The listing builds one solid part. Answer for the finished solid, in the listing's coordinates (mm). A direction names the side the tool comes from. Round coordinates to 2 decimals unless told otherwise and drop trailing zeros. Write each loop counter-clockwise with the first axis right and the second up, starting at its lowest first coordinate (ties: lowest second). Pieces come first, ordered by that corner, then holes.
Item 1: Each of these flat-tipped pins is pushed along its axis until it touches: pin 1 (8 mm diameter, centred on y = -8, z = 5, fed in from -X); pin 2 (1.5 mm diameter, centred on y = 12, z = 5, fed in from -X); pin 3 (6 mm diameter, centred on x = -1, z = 10, fed in from +Y) (3 decimals); pin 4 (4 mm diameter, centred on x = -11.5, z = 4, fed in from -Y). Where does it stop, or does it pass through?
Item 2: A tool of negligible diameter and unlimited length cuts with its end or side. For faces 5 (the face through (-5.474, 3.219, 12.522)), 6 (the face through (-15.12, -11.59, 26.97)), 7 (the face through (4, 9, 3.175)), 8 (the face through (0, 0, 28.575)), 9 (the face through (-0.21, 15.57, 26.97)), from which of +Z, -Z, +X, -X, +Y, -Y can it reach the whole face along a straight path? Write none if from no direction.
Item 3: For a pull along X with two mould halves and no side action, classify faces 1 (the face through (5.525, 3.131, 12.522)), 2 (the face through (-15.12, -11.59, 1.57)), 3 (the face through (-5.525, -3.131, 12.522)), 4 (the face through (-9, -4, 25.4)) as +X half, -X half, draft (parallel to the pull), parting line (faces both ways), or undercut.
Item 4: Find section A-A on x = 0. Give the vertices of the cut face in (y, z) (3 decimals).
Item 5: Find section C-C on y = 3. Give the vertices of the cut face in (x, z) (3 decimals).
Item 6: Find section B-B on z = 23.5. Give the vertices of the cut face in (x, y) (3 decimals), then the cut area to 3 significant figures.
Item 7: Find the intervals of material crossed by probe 1 along Z at (x, y) = (-12, 2) (3 decimals); probe 2 along Y at (x, z) = (0, 26.95); probe 3 along X at (y, z) = (-6, 16), in increasing order.
Item 8: Find section D-D on x = 14. Give the vertices of the cut face in (y, z) (3 decimals).
```python
from build123d import *

# Parameters (mm, degrees)
SKETCH1_R           = 19.05
BOSS_EXTRUDE1_DEPTH = 3.175
SKETCH2_R           = 9.525
BOSS_EXTRUDE2_DEPTH = 22.225
SKETCH3_R           = 19.05
SKETCH3_R_2         = 1.5875
BOSS_EXTRUDE3_DEPTH = 3.175


with BuildPart() as part:
    # Sketch1 → Boss-Extrude1 (new body)
    with BuildSketch(Plane.XY):
        Circle(SKETCH1_R)
        Polygon((7.332348419, 0), (3.666174209, 6.35), (-3.666174209, 6.35), (-7.332348419, 0), (-3.666174209, -6.35), (3.666174209, -6.35), align=None, mode=Mode.SUBTRACT)
    extrude(amount=BOSS_EXTRUDE1_DEPTH)

    # Sketch2 → Boss-Extrude2 (add)
    with BuildSketch(Plane.XY.offset(3.175)):
        Circle(SKETCH2_R)
        Polygon((7.332348419, 0), (3.666174209, 6.35), (-3.666174209, 6.35), (-7.332348419, 0), (-3.666174209, -6.35), (3.666174209, -6.35), align=None, mode=Mode.SUBTRACT)
    extrude(amount=BOSS_EXTRUDE2_DEPTH)

    # Sketch3 → Boss-Extrude3 (add)
    with BuildSketch(Plane.XY.offset(25.4)):
        Circle(SKETCH3_R)
        with Locations((0, 13.995802971)):
            Circle(SKETCH3_R_2, mode=Mode.SUBTRACT)
    extrude(amount=BOSS_EXTRUDE3_DEPTH)


solid = part.part
```
Check values:
1. pin 1: stops at x = -18.53
1. pin 2: passes through
1. pin 3: stops at y = 9.525
1. pin 4: stops at y = -16.41
2. face 5: -Z
2. face 6: +Z, -Z
2. face 7: none
2. face 8: +Z, +X, -X, +Y, -Y
2. face 9: +Z
3. face 1: undercut
3. face 2: parting line
3. face 3: undercut
3. face 4: draft
4. outline: (-19.05, 0) - (-6.35, 0) - (-6.35, 25.4) - (6.35, 25.4) - (6.35, 0) - (19.05, 0) - (19.05, 3.175) - (9.525, 3.175) - (9.525, 25.4) - (12.408, 25.4) - (12.408, 28.575) - (-19.05, 28.575) - (-19.05, 25.4) - (-9.525, 25.4) - (-9.525, 3.175) - (-19.05, 3.175) - close; (15.583, 25.4) - (19.05, 25.4) - (19.05, 28.575) - (15.583, 28.575) - close
5. outline: (-18.812, 0) - (-5.6, 0) - (-5.6, 25.4) - (5.6, 25.4) - (5.6, 0) - (18.812, 0) - (18.812, 3.175) - (9.04, 3.175) - (9.04, 25.4) - (18.812, 25.4) - (18.812, 28.575) - (-18.812, 28.575) - (-18.812, 25.4) - (-9.04, 25.4) - (-9.04, 3.175) - (-18.812, 3.175) - close
6. outline: circle Ø19.05 at (0, 0); hole (-7.332, 0) - (-3.666, -6.35) - (3.666, -6.35) - (7.332, 0) - (3.666, 6.35) - (-3.666, 6.35) - close
6. area: 145 mm2
7. probe 1: z = 0 to 3.175, 25.4 to 28.575
7. probe 2: y = -19.05 to 12.41, 15.58 to 19.05
7. probe 3: x = -7.4 to -3.87, 3.87 to 7.4
8. outline: (-12.919, 0) - (12.919, 0) - (12.919, 3.175) - (-12.919, 3.175) - close; (-12.919, 25.4) - (12.919, 25.4) - (12.919, 28.575) - (-12.919, 28.575) - close
